Work out the finished part from the listing and answer in its coordinate system (mm). Face numbers are marked on the shaded views. Give positions to 0.01 mm unless a question says otherwise; leave off trailing zeros. Write each loop counter-clockwise with the first axis right and the second up, starting at its lowest first coordinate (ties: lowest second). Pieces come first, ordered by that corner, then holes. Notation, with made-up numbers: (5.5, -40) - (47.5, -40) arc R10 ccw to (47.5, -23) - close; hole circle Ø4 at (7.25, -36). An arc over 180 degrees is marked (long way). Write item = value, one per line.
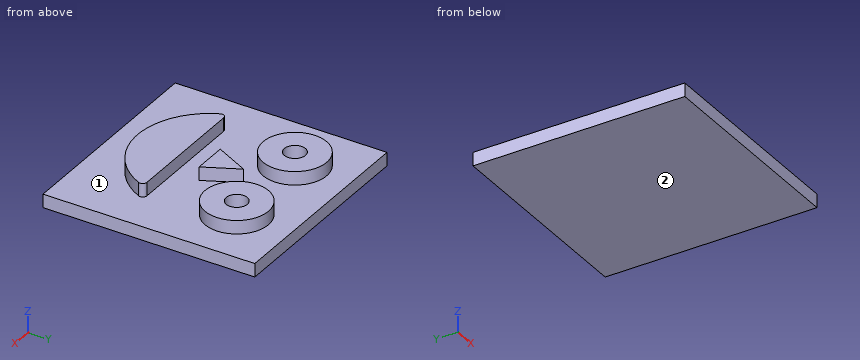
from build123d import *

# Parameters (mm, degrees)
SKETCH1_W           = 50
SKETCH1_H           = 50
BOSS_EXTRUDE1_DEPTH = 3.175
SKETCH2_R           = 7.5
SKETCH2_R_2         = 2.5
BOSS_EXTRUDE2_DEPTH = 3.175
FILLET1_R           = 1


with BuildPart() as part:
    # Sketch1 → Boss-Extrude1 (new body)
    with BuildSketch(Plane.XY):
        Rectangle(SKETCH1_W, SKETCH1_H)
    extrude(amount=BOSS_EXTRUDE1_DEPTH)

    # Sketch2 → Boss-Extrude2 (add)
    with BuildSketch(Plane.XY.offset(3.175)):
        with Locations((-11, 12)):
            Circle(SKETCH2_R)
        with Locations((-11, 12)):
            Circle(SKETCH2_R_2, mode=Mode.SUBTRACT)
        with Locations((11, 12)):
            Circle(SKETCH2_R)
        with Locations((11, 12)):
            Circle(SKETCH2_R_2, mode=Mode.SUBTRACT)
        with BuildLine():
            Line((-16, -7), (16, -7))
            ThreePointArc((16, -7), (0, -18.255437353), (-16, -7))
        make_face()
        Polygon((0, 6.744562647), (4, -1.255437353), (-4, -1.255437353), align=None)
    extrude(amount=BOSS_EXTRUDE2_DEPTH)

    # Fillet1
    fillet1_edges = [part.edges().sort_by_distance(p)[0] for p in [
        (-16, -7, 4.7625),
        (16, -7, 4.7625),
    ]]
    fillet(fillet1_edges, radius=FILLET1_R)


solid = part.part
1. Find section B-B, the plane y = 12. Give the vertices of the cut face in (x, z) (3 decimals).
Solution:
outline = (-25, 0) - (25, 0) - (25, 3.175) - (18.5, 3.175) - (18.5, 6.35) - (13.5, 6.35) - (13.5, 3.175) - (8.5, 3.175) - (8.5, 6.35) - (3.5, 6.35) - (3.5, 3.175) - (-3.5, 3.175) - (-3.5, 6.35) - (-8.5, 6.35) - (-8.5, 3.175) - (-13.5, 3.175) - (-13.5, 6.35) - (-18.5, 6.35) - (-18.5, 3.175) - (-25, 3.175) - close
2. Find section A-A, the plane z = 4. Give the vertices of the cut face in (x, y).
Solution:
outline = circle Ø15 at (-11, 12); (-15.42, -8.42) arc R17 ccw to (15.42, -8.42) arc R1 ccw to (14.51, -7) - (-14.51, -7) arc R1 ccw to start; (-4, -1.26) - (4, -1.26) - (0, 6.74) - close; circle Ø15 at (11, 12); hole circle Ø5 at (-11, 12); hole circle Ø5 at (11, 12)
3. Find section D-D, the plane x = 11. Give the vertices of the cut face in (y, z) (3 decimals), then the cut area to 3 significant figures.
Solution:
outline = (-25, 0) - (25, 0) - (25, 3.175) - (19.5, 3.175) - (19.5, 6.35) - (14.5, 6.35) - (14.5, 3.175) - (9.5, 3.175) - (9.5, 6.35) - (4.5, 6.35) - (4.5, 3.175) - (-7, 3.175) - (-7, 6.35) - (-14.217, 6.35) - (-14.217, 3.175) - (-25, 3.175) - close
area = 213 mm^2
4. Straight lines are drawn through the part: line 1 (X direction, y = 11, z = 4.5); line 2 (Y direction, x = -11, z = 4.8); line 3 (Z direction, x = 7, y = 5) (3 decimals). For each, find the intervals that lie inside material, in ascending order.
Solution:
line_1 = -18.43 to -13.29, -8.71 to -3.57, 3.57 to 8.71, 13.29 to 18.43
line_2 = -14.22 to -7, 4.5 to 9.5, 14.5 to 19.5
line_3 = 0 to 3.175
5. Given pin 1 (1.5 mm diameter, centred on x = -10.5, y = 11.5, fed in from +Z) (3 decimals); pin 2 (2.5 mm diameter, centred on x = 12, y = 13, fed in from +Z); pin 3 (2.5 mm diameter, centred on x = 3.5, z = 5.5, fed in from +Y); pin 4 (1.5 mm diameter, centred on y = -3.5, z = 5, fed in from +X), each flat-ended and moving along its own axis, determine where each tip first touches the part or whether it passes through.
Solution:
pin_1 = 3.175
pin_2 = 6.35
pin_3 = 16.15
pin_4 = through
6. Find section C-C, the plane x = -5.5. Give the vertices of the cut face in (y, z) (3 decimals), then the cut area to 3 significant figures.
Solution:
outline = (-25, 0) - (25, 0) - (25, 3.175) - (17.099, 3.175) - (17.099, 6.35) - (6.901, 6.35) - (6.901, 3.175) - (-7, 3.175) - (-7, 6.35) - (-17.341, 6.35) - (-17.341, 3.175) - (-25, 3.175) - close
area = 224 mm^2
7. For a pull along Y with two mould halves and no side action, classify the marked faces 1 and 2 as pulls with the +Y half, pulls with the -Y half, needs draft (parallel to the pull), parting line crosses it, or undercut.
Solution:
face_1 = undercut
face_2 = needs draft
